from build123d import *

# Parameters (mm, degrees)
SKETCH004_R      = 1.75
SKETCH004_W      = 4
SKETCH004_H      = 27
PAD_DEPTH        = 3
PAD006_DEPTH     = 3
PAD007_DEPTH     = 3
SKETCH_R         = 1.75
PAD008_DEPTH     = 3
SKETCH003007_R   = 1.75
PAD010_DEPTH     = 3
SKETCH002_W      = 48
SKETCH002_H      = 3
PAD003_DEPTH     = 3
SKETCH003004_R   = 1.75
PAD009_DEPTH     = 3
SKETCH003003_W   = 240
SKETCH003003_H   = 100
SKETCH003003_R   = 1.75
SKETCH003003_W_2 = 3
SKETCH003003_H_2 = 9.6
SKETCH003003_W_3 = 14.6
SKETCH003003_H_3 = 3
PAD001_DEPTH     = 3
FILLET_R         = 5
FILLET001_R      = 1


with BuildPart() as pad:
    # Sketch004 → Pad (new body)
    with BuildSketch(Plane.XY):
        with Locations((60, -17.5)):
            Circle(SKETCH004_R)
        with Locations((60, 17.5)):
            Circle(SKETCH004_R)
        with Locations((95, 17.5)):
            Circle(SKETCH004_R)
        with Locations((95, -17.5)):
            Circle(SKETCH004_R)
        with Locations((65, 0)):
            Rectangle(SKETCH004_W, SKETCH004_H)
    extrude(amount=PAD_DEPTH)


with BuildPart() as pad006:
    # Sketch003006 → Pad006 (new body)
    with BuildSketch(Plane.XY):
        with BuildLine():
            ThreePointArc((97.625206, 30.21875), (100, 23), (102.374794, 30.21875))
            ThreePointArc((102.374794, 30.21875), (100, 33.5), (97.625206, 30.21875))
        make_face()
    extrude(amount=PAD006_DEPTH)


with BuildPart() as pad007:
    # Sketch003005 → Pad007 (new body)
    with BuildSketch(Plane.XY):
        with BuildLine():
            ThreePointArc((-102.374794, 30.21875), (-100, 23), (-97.625206, 30.21875))
            ThreePointArc((-97.625206, 30.21875), (-100, 33.5), (-102.374794, 30.21875))
        make_face()
    extrude(amount=PAD007_DEPTH)


with BuildPart() as pad008:
    # Sketch → Pad008 (new body)
    with BuildSketch(Plane.XY):
        with Locations((-90, 30)):
            Circle(SKETCH_R)
        with Locations((-60, 30)):
            Circle(SKETCH_R)
        with Locations((-90, 0)):
            Circle(SKETCH_R)
        with Locations((-60, 0)):
            Circle(SKETCH_R)
        with Locations((-80, 0)):
            Circle(SKETCH_R)
        with Locations((-80, 25)):
            Circle(SKETCH_R)
        with Locations((-60, 25)):
            Circle(SKETCH_R)
        with Locations((-70, 0)):
            Circle(SKETCH_R)
        with Locations((-70, 20)):
            Circle(SKETCH_R)
        with Locations((-60, 20)):
            Circle(SKETCH_R)
    extrude(amount=PAD008_DEPTH)


with BuildPart() as pad010:
    # Sketch003007 → Pad010 (new body)
    with BuildSketch(Plane.XY):
        with Locations((-108.5, 38.5)):
            Circle(SKETCH003007_R)
        with Locations((-108.5, -38.5)):
            Circle(SKETCH003007_R)
        with Locations((108.5, -38.5)):
            Circle(SKETCH003007_R)
        with Locations((108.5, 38.5)):
            Circle(SKETCH003007_R)
    extrude(amount=PAD010_DEPTH)


with BuildPart() as pad003:
    # Sketch002 → Pad003 (new body)
    with BuildSketch(Plane.XY):
        with Locations((0, 34.5)):
            Rectangle(SKETCH002_W, SKETCH002_H)
        with Locations((0, -26.5)):
            Rectangle(SKETCH002_W, SKETCH002_H)
    extrude(amount=PAD003_DEPTH)


with BuildPart() as pad009:
    # Sketch003004 → Pad009 (new body)
    with BuildSketch(Plane.XY):
        with Locations((-90, -40)):
            Circle(SKETCH003004_R)
        with Locations((-60, -40)):
            Circle(SKETCH003004_R)
        with Locations((-90, -10)):
            Circle(SKETCH003004_R)
        with Locations((-60, -10)):
            Circle(SKETCH003004_R)
        with Locations((-80, -10)):
            Circle(SKETCH003004_R)
        with Locations((-80, -35)):
            Circle(SKETCH003004_R)
        with Locations((-60, -35)):
            Circle(SKETCH003004_R)
        with Locations((-70, -10)):
            Circle(SKETCH003004_R)
        with Locations((-70, -30)):
            Circle(SKETCH003004_R)
        with Locations((-60, -30)):
            Circle(SKETCH003004_R)
    extrude(amount=PAD009_DEPTH)


with BuildPart() as fillet001:
    # Sketch003003 → Pad001 (new body)
    with BuildSketch(Plane.XY):
        Rectangle(SKETCH003003_W, SKETCH003003_H)
        with Locations((93.5, -32.8)):
            Circle(SKETCH003003_R, mode=Mode.SUBTRACT)
        with Locations((108.5, -25)):
            Rectangle(SKETCH003003_W_2, SKETCH003003_H_2, mode=Mode.SUBTRACT)
        with Locations((108.5, 25)):
            Rectangle(SKETCH003003_W_2, SKETCH003003_H_2, mode=Mode.SUBTRACT)
        with Locations((-108.5, 25)):
            Rectangle(SKETCH003003_W_2, SKETCH003003_H_2, mode=Mode.SUBTRACT)
        with Locations((-108.5, -25)):
            Rectangle(SKETCH003003_W_2, SKETCH003003_H_2, mode=Mode.SUBTRACT)
        with Locations((-77.5, 38.5)):
            Rectangle(SKETCH003003_W_3, SKETCH003003_H_3, mode=Mode.SUBTRACT)
        with Locations((-32.5, 38.5)):
            Rectangle(SKETCH003003_W_3, SKETCH003003_H_3, mode=Mode.SUBTRACT)
        with Locations((32.5, 38.5)):
            Rectangle(SKETCH003003_W_3, SKETCH003003_H_3, mode=Mode.SUBTRACT)
        with Locations((77.5, 38.5)):
            Rectangle(SKETCH003003_W_3, SKETCH003003_H_3, mode=Mode.SUBTRACT)
    extrude(amount=PAD001_DEPTH)

    # Cut: cut Pad009
    add(pad009.part, mode=Mode.SUBTRACT)

    # Cut001: cut Pad003
    add(pad003.part, mode=Mode.SUBTRACT)

    # Cut002: cut Pad010
    add(pad010.part, mode=Mode.SUBTRACT)

    # Cut003: cut Pad008
    add(pad008.part, mode=Mode.SUBTRACT)

    # Cut004: cut Pad007
    add(pad007.part, mode=Mode.SUBTRACT)

    # Cut005: cut Pad006
    add(pad006.part, mode=Mode.SUBTRACT)

    # Cut006: cut Pad
    add(pad.part, mode=Mode.SUBTRACT)

    # Fillet
    fillet_edges = [fillet001.edges().sort_by_distance(p)[0] for p in [
        (-120, 50, 1.5),
        (120, 50, 1.5),
        (-120, -50, 1.5),
        (120, -50, 1.5),
    ]]
    fillet(fillet_edges, radius=FILLET_R)

    # Fillet001
    fillet001_edges = [fillet001.edges().sort_by_distance(p)[0] for p in [
        (-24, -28, 1.5),
        (-24, -25, 1.5),
        (24, -28, 1.5),
        (24, -25, 1.5),
        (-24, 33, 1.5),
        (-24, 36, 1.5),
        (24, 33, 1.5),
        (24, 36, 1.5),
        (63, -13.5, 1.5),
        (63, 13.5, 1.5),
        (67, -13.5, 1.5),
        (67, 13.5, 1.5),
    ]]
    fillet(fillet001_edges, radius=FILLET001_R)


solid = fillet001.part
Model file for the job. Use its own axes, mm. Give positions to 0.01 mm unless a question says otherwise; leave off trailing zeros. Loops run counter-clockwise (first coordinate to the right, second up) from the corner with the lowest first, then second, coordinate; pieces in that order, holes last. Notation, with made-up numbers: (-12.5, 27.25) - (8.5, 27.25) arc R25 cw to (8.5, 49.25) - close; hole circle Ø3 at (18, 15). An arc over 180 degrees is marked (long way). Use one line per item in the form item = value.
(1) Cut at D-D (z = 1.9). Count the separate pieces of the cut face and the enclosed holes in it, then the cut area to 3 significant figures.
Determined:
separate_pieces = 1
enclosed_holes = 42
area = 22,900 mm^2
(2) Drill centre lines: L1, parallel to X at y = -27, z = 1.4; L2, parallel to Y at x = 19, z = 0.9; L3, parallel to Y at x = -90, z = 1.75. Where is each one in solid material? Low to high.
Determined:
L1 = -120 to -110, -107 to -24, 24 to 107, 110 to 120
L2 = -50 to -28, -25 to 33, 36 to 50
L3 = -50 to -41.75, -38.25 to -11.75, -8.25 to -1.75, 1.75 to 28.25, 31.75 to 50
(3) Pull direction X, two halves, no side cores. Call faces 1 (the face through (118, 49, 2)), 2 (the face through (-119, 48, 2)), 3 (the face through (100, 23, 1)): pulls with the +X half, pulls with the -X half, needs draft (parallel to the pull), parting line crosses it, or undercut.
Determined:
face_1 = pulls with the +X half
face_2 = pulls with the -X half
face_3 = undercut
(4) Cut at C-C (x = -100). Give the cut face in (y, z).
Determined:
outline = (-50, 0) - (23, 0) - (23, 3) - (-50, 3) - close; (33.5, 0) - (50, 0) - (50, 3) - (33.5, 3) - close
(5) Drop a flat-ended pin along its axis: P1, Ø2, axis at x = -90, y = -40, coming from the +Z side. Give the stop position or say it passes through.
Determined:
P1 = through
(6) Cut at A-A (x = -16). Give the cut face in (y, z).
Determined:
outline = (-50, 0) - (-28, 0) - (-28, 3) - (-50, 3) - close; (-25, 0) - (33, 0) - (33, 3) - (-25, 3) - close; (36, 0) - (50, 0) - (50, 3) - (36, 3) - close
(7) Cut at B-B (y = 4). Give the cut face in (x, z).
Determined:
outline = (-120, 0) - (63, 0) - (63, 3) - (-120, 3) - close; (67, 0) - (120, 0) - (120, 3) - (67, 3) - close
